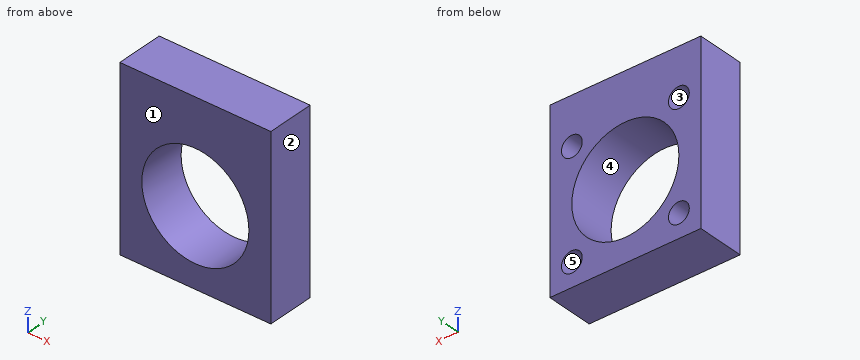
```python
from build123d import *

# Parameters (mm, degrees)
F0_W     = 12.7
F0_H     = 15
F0_R     = 4.5
F1_DEPTH = 4
F2_D     = 1.75
F2_DEPTH = 2
F2_TIP   = 0.5257530416
F3_D     = 1.75
F3_DEPTH = 2
F3_TIP   = 0.5257530416


with BuildPart() as f1:
    # F0 (on Front) → F1 (new body)
    with BuildSketch(Plane.XZ):
        with Locations((0, 1)):
            Rectangle(F0_W, F0_H)
        Circle(F0_R, mode=Mode.SUBTRACT)
    extrude(amount=F1_DEPTH)

    # F2
    with Locations(Plane(origin=(0, 0, 0), x_dir=(1, 0, 0), z_dir=(0, 1, 0))):
        with Locations((-4.5, -4.5)):
            Hole(F2_D / 2, depth=F2_DEPTH)
            with Locations((0, 0, -(F2_DEPTH + F2_TIP / 2))):  # 118° drill point
                Cone(0, F2_D / 2, F2_TIP, mode=Mode.SUBTRACT)

    # F3
    with Locations(Plane(origin=(0, 0, 0), x_dir=(1, 0, 0), z_dir=(0, 1, 0))):
        with Locations((4.5, -4.5), (4.5, 4.5), (-4.5, 4.5)):
            Hole(F3_D / 2, depth=F3_DEPTH)
            with Locations((0, 0, -(F3_DEPTH + F3_TIP / 2))):  # 118° drill point
                Cone(0, F3_D / 2, F3_TIP, mode=Mode.SUBTRACT)


solid = f1.part
```
Geometry: final body of the model. Coordinates: model frame, mm. Face numbers are marked on the shaded views. A direction names the side the tool comes from. Coordinates: 2 decimals unless noted, no trailing zeros. Order: outer loops, then holes, each group sorted by start corner. A loop starts at its lowest first (then second) coordinate and runs counter-clockwise, first axis right, second up. Notation, with made-up numbers: (-24, 57) -> (9, 57) arc R34 ccw to (9, 95) -> close; hole circle Ø10 at (55, 31). An arc over 180 degrees is marked (long way). Write each question's results on one line, items separated by ' | '. Start each with the question number.
1) Material intervals for line 1 along Z through (x, y) = (4.75, -0.25); line 2 along X through (y, z) = (-3.15, -1.25); line 3 along X through (y, z) = (-0.4, 3.5), sorted ascending.
2) First-contact query: pin 1 (1.6 mm diameter, centred on x = 4.5, z = -4.5, fed in from +Y). Flat tip, straight axial feed; report the tip coordinate or a pass-through.
3) Mould query, pull axis X, two halves, no side actions, for the marked faces 1, 2 and 3. Classes: released by +X, released by -X, zero draft, split by the parting line, or undercut.
4) Set-up query: the marked faces 4 and 5. Return all of +Z, -Z, +X, -X, +Y, -Y with unobstructed straight access to the full face (end or side cutting, diameter ignored); none if empty.
5) Cut plane A-A, the plane z = 0. Output: boundary loops of the cut face in (x, y).
6) Cut plane D-D, the plane y = -3. Output: boundary loops of the cut face in (x, z), and give its area (3 significant figures).
7) Cut plane C-C, the plane y = -1.45. Output: boundary loops of the cut face in (x, z) (3 decimals).
8) Cut plane B-B, the plane x = 0. Output: boundary loops of the cut face in (y, z).
Checks:
1) line 1: -6.5 to -5.34, -3.66 to 3.66, 5.34 to 8.5 | line 2: -6.35 to -4.32, 4.32 to 6.35 | line 3: -6.35 to -2.83, 2.83 to 6.35
2) pin 1: y = -2.05
3) face 1: zero draft | face 2: released by +X | face 3: undercut
4) face 4: +Y, -Y | face 5: +Y
5) outline: (-6.35, -4) -> (-4.5, -4) -> (-4.5, 0) -> (-6.35, 0) -> close; (4.5, -4) -> (6.35, -4) -> (6.35, 0) -> (4.5, 0) -> close
6) outline: (-6.35, -6.5) -> (6.35, -6.5) -> (6.35, 8.5) -> (-6.35, 8.5) -> close; hole circle Ø9 at (0, 0) | area: 127 mm^2
7) outline: (-6.35, -6.5) -> (6.35, -6.5) -> (6.35, 8.5) -> (-6.35, 8.5) -> close; hole circle Ø1.75 at (-4.5, -4.5); hole circle Ø1.75 at (-4.5, 4.5); hole circle Ø9 at (0, 0); hole circle Ø1.75 at (4.5, -4.5); hole circle Ø1.75 at (4.5, 4.5)
8) outline: (-4, -6.5) -> (0, -6.5) -> (0, -4.5) -> (-4, -4.5) -> close; (-4, 4.5) -> (0, 4.5) -> (0, 8.5) -> (-4, 8.5) -> close
